Input: part model. Units: mm. Frame: model coordinates. A direction names the side the tool comes from. Give positions to 0.01 mm unless a question says otherwise; leave off trailing zeros. Order: outer loops, then holes, each group sorted by start corner. A loop starts at its lowest first (then second) coordinate and runs counter-clockwise, first axis right, second up. Notation, with made-up numbers: M 62.25,-24 L 99.25,-24 A14 cw 99.25,-14 Z; hole C -36.75,26 d9. An arc over 180 degrees is marked long. Use a Markdown table: item, result.
from build123d import *

# Parameters (mm, degrees)
F0_R     = 24
F0_R_2   = 6.5
F1_DEPTH = 3
F0_R_3   = 5
F2_DEPTH = 25
F3_R     = 7


# Not quite as in the source:
# - a fillet or chamfer that OpenCascade refuses, or shapes differently, is made with other operations: its cross-section is extruded or revolved along the edge and cut away or added


with BuildPart() as f1:
    # F0 (on Top) → F1 (new body)
    with BuildSketch(Plane.XY):
        Circle(F0_R)
        Circle(F0_R_2, mode=Mode.SUBTRACT)
    extrude(amount=F1_DEPTH)

    # F0 (on Top) → F2 (join)
    with BuildSketch(Plane.XY):
        Circle(F0_R_2)
        Circle(F0_R_3, mode=Mode.SUBTRACT)
    extrude(amount=F2_DEPTH)

    # F3
    f3_edges = [f1.edges().sort_by_distance(p)[0] for p in [
        (-5, 0, 0),
    ]]
    fillet(f3_edges, radius=F3_R)

    # F4: fillet of radius 4.104163056 on 1 edges, made by hand

    # F4_s1 → F4_t2 (revolve, cut)
    with BuildSketch(Plane.XZ):
        with BuildLine():
            ThreePointArc((20.0471556651, 0), (22.5283337288, 0.8349261716), (24, 3))
            Line((24, 3), (24, 0))
            Line((24, 0), (20.0471556651, 0))
        make_face()
    revolve(axis=Axis((0, 0, 0), (0, 0, 1)), mode=Mode.SUBTRACT)


solid = f1.part
1) First-contact query: pin 1 Ø4 at (x, z) = (1.5, 15) entering from -Y; pin 2 Ø3 at (x, z) = (-3.5, 9) entering from +Y; pin 3 Ø12 at (x, y) = (-16.5, -18.5) entering from +Z; pin 4 Ø8 at (x, y) = (0, 0) entering from +Z. Flat tips, straight axial feed; report the tip coordinate or a pass-through.
Response values:
| item | result |
|---|---|
| pin 1 | stops at y = -6.5 |
| pin 2 | stops at y = 6.18 |
| pin 3 | stops at z = 3 |
| pin 4 | passes through |
2) Material intervals for line 1 (Z direction, x = 12, y = -5); line 2 (Y direction, x = 0, z = 19.5); line 3 (X direction, y = -2, z = 6.25), sorted ascending. Write a range as from..to.
Response values:
| item | result |
|---|---|
| line 1 | z = 0..3 |
| line 2 | y = -6.5..-5, 5..6.5 |
| line 3 | x = -6.18..-4.63, 4.63..6.18 |
3) Cut plane C-C on z = 11. Return loops of the section in (x, y).
Response values:
| item | result |
|---|---|
| outline | C 0,0 d13; hole C 0,0 d10 |
4) Reachability of faces 1 (the face through (5, -5, 3)), 2 (the face through (2, -5, 25)) from +Z, -Z, +X, -X, +Y, -Y: full face, straight path, thin tool, end or side. Return the list, or none.
Response values:
| item | result |
|---|---|
| face 1 | +Z |
| face 2 | +Z, +X, -X, +Y, -Y |
5) Cut plane A-A on x = 0. Return loops of the section in (y, z).
Response values:
| item | result |
|---|---|
| outline | M -24,3 A4.1 ccw -20.05,0 L -12,0 A7 ccw -5,7 L -5,25 L -6.5,25 L -6.5,3 Z; M 5,7 A7 ccw 12,0 L 20.05,0 A4.1 ccw 24,3 L 6.5,3 L 6.5,25 L 5,25 Z |
